from build123d import *

# Parameters (mm, degrees)
F0_W     = 5.4
F0_H     = 0.3
F1_DEPTH = 4
F0_H_2   = 2.85
F2_DEPTH = 0.2


with BuildPart() as f1:
    # F0 (on Front) → F1 (new body)
    with BuildSketch(Plane.XZ):
        Polygon((-3, 12.9), (-3, 0), (-2.7, 0), (-2.7, 0.3), (-2.7, 3.15), (-2.7, 3.45), (-2.7, 6.3), (-2.7, 6.6), (-2.7, 9.45), (-2.7, 9.75), (-2.7, 12.6), (-2.7, 12.9), align=None)
        Polygon((2.7, 0.3), (2.7, 0), (3, 0), (3, 12.9), (2.7, 12.9), (2.7, 12.6), (2.7, 9.75), (2.7, 9.45), (2.7, 6.6), (2.7, 6.3), (2.7, 3.45), (2.7, 3.15), align=None)
        with Locations((0, 12.75)):
            Rectangle(F0_W, F0_H)
        with Locations((0, 9.6)):
            Rectangle(F0_W, F0_H)
        with Locations((0, 6.45)):
            Rectangle(F0_W, F0_H)
        with Locations((0, 3.3)):
            Rectangle(F0_W, F0_H)
        with Locations((0, 0.15)):
            Rectangle(F0_W, F0_H)
    extrude(amount=F1_DEPTH)

    # F0 (on Front) → F2 (join)
    with BuildSketch(Plane.XZ):
        with Locations((0, 11.175)):
            Rectangle(F0_W, F0_H_2)
        with Locations((0, 4.875)):
            Rectangle(F0_W, F0_H_2)
        with Locations((0, 1.725)):
            Rectangle(F0_W, F0_H_2)
        with Locations((0, 8.025)):
            Rectangle(F0_W, F0_H_2)
    extrude(amount=F2_DEPTH)


solid = f1.part
CAD build for the part. Positions are in the model's coordinates, mm. A direction names the side the tool comes from. Round coordinates to 2 decimals unless told otherwise and drop trailing zeros. Order: outer loops, then holes, each group sorted by start corner. A loop starts at its lowest first (then second) coordinate and runs counter-clockwise, first axis right, second up. Notation, with made-up numbers: (17.5, -18.5) - (73.5, -18.5) arc R29 cw to (73.5, 19.5) - close; hole circle Ø10 at (9.25, 17.25). An arc over 180 degrees is marked (long way). Return JSON: item names as keys, results as strings.
(1) Wall check: probe 1 along Z at (x, y) = (1.55, -1.2); probe 2 along X at (y, z) = (-1.05, 12.25). Give the ranges that are in metal, low to high. Write a range as from..to.
Answer key:
{"probe 1": "z = 0..0.3, 3.15..3.45, 6.3..6.6, 9.45..9.75, 12.6..12.9", "probe 2": "x = -3..-2.7, 2.7..3"}
(2) Pull direction Z, two halves, no side cores. Call faces 3 (the face through (3, -2, 6)), 4 (the face through (0, -2, 6.6)), 5 (the face through (0, -2, 0)): +Z half, -Z half, draft (parallel to the pull), parting line (faces both ways), or undercut.
Answer key:
{"face 3": "draft", "face 4": "undercut", "face 5": "-Z half"}
(3) Cut at B-B (x = -0.4). Give the cut face in (y, z).
Answer key:
{"outline": "(-4, 0) - (0, 0) - (0, 12.9) - (-4, 12.9) - (-4, 12.6) - (-0.2, 12.6) - (-0.2, 9.75) - (-4, 9.75) - (-4, 9.45) - (-0.2, 9.45) - (-0.2, 6.6) - (-4, 6.6) - (-4, 6.3) - (-0.2, 6.3) - (-0.2, 3.45) - (-4, 3.45) - (-4, 3.15) - (-0.2, 3.15) - (-0.2, 0.3) - (-4, 0.3) - close"}
(4) Cut at C-C (z = 1). Give the cut face in (x, y).
Answer key:
{"outline": "(-3, -4) - (-2.7, -4) - (-2.7, -0.2) - (2.7, -0.2) - (2.7, -4) - (3, -4) - (3, 0) - (-3, 0) - close"}
(5) Tool access for faces 1 (the face through (0, -2, 6.3)), 2 (the face through (-3, -2, 7)): list every direction of +Z, -Z, +X, -X, +Y, -Y with a clear straight run to the whole face (end or side of a thin tool).
Answer key:
{"face 1": "-Y", "face 2": "+Z, -Z, -X, +Y, -Y"}
(6) Cut at A-A (y = -3.5). Give the cut face in (x, z), then the cut area to 3 significant figures.
Answer key:
{"outline": "(-3, 0) - (3, 0) - (3, 12.9) - (-3, 12.9) - close; hole (-2.7, 0.3) - (2.7, 0.3) - (2.7, 3.15) - (-2.7, 3.15) - close; hole (-2.7, 3.45) - (2.7, 3.45) - (2.7, 6.3) - (-2.7, 6.3) - close; hole (-2.7, 6.6) - (2.7, 6.6) - (2.7, 9.45) - (-2.7, 9.45) - close; hole (-2.7, 9.75) - (2.7, 9.75) - (2.7, 12.6) - (-2.7, 12.6) - close", "area": "15.8 mm^2"}
(7) Pin check, flat tips, straight feed: pin 1 Ø1 at (x, y) = (1.5, -3.5) entering from -Z; pin 2 Ø1 at (x, z) = (1.5, 8.5) entering from -Y. Stop position of each tip, or through.
Answer key:
{"pin 1": "stops at z = 0", "pin 2": "stops at y = -0.2"}
